Autodesk Inventor part; units mm, degrees
ref_plane "YZ Plane" through (0, 0, 0) normal (1, 0, 0) x (0, 1, 0)
ref_plane "XZ Plane" through (0, 0, 0) normal (0, 1, 0) x (-1, 0, 0)
ref_plane "XY Plane" through (0, 0, 0) normal (0, 0, 1) x (1, 0, 0)
sketch "Sketch1" plane through (0, 0, 0) normal (0, 0, 1) x (1, 0, 0)
  line L0 (-70, -100) -> (70, -100)
  line L1 (70, -100) -> (70, 100)
  line L2 (70, 100) -> (-70, 100)
  line L3 (-70, 100) -> (-70, -100)
  line L4 (-70, -100) -> (70, 100) construction
  line L5 (70, -100) -> (-70, 100) construction
  point P0 (0, 0)
  dimension "d154" = 140
  dimension "d155" = 200
extrude "Plate5" add sketch "Sketch1" along normal blind 2
sketch "Sketch7" plane through (68, -100, 2) normal (1, 0, 0) x (0, 1, 0)
  line L0 (200, 0) -> (0, 0)
  line L1 (0, 0) -> (0, -30)
  line L2 (0, -30) -> (200, -30)
  line L3 (200, -30) -> (200, 0)
edge flange "Flange3" height 30 angle 90 thickness 2 bend radius 2.75 thickness toward (1, 0, 0) relief round relief width 2 relief depth 1 corner gap 2.75 corner form 0 edges at (70, 0, 0) (-70, 0, 0) wall of the first edge with corners at (68, 100, 2) (68, -100, 2) (68, -100, -28) (68, 100, -28)
bend "Bend3"
corner "Corner3"
sketch "Sketch8" plane through (-68, -100, -26) normal (0, 0, -1) x (-1, 0, 0)
  line L0 (0, 200) -> (0, 0)
  line L1 (0, 0) -> (35, 0)
  line L2 (35, 0) -> (35, 200)
  line L3 (35, 200) -> (0, 200)
edge flange "Flange4" height 35 angle 90 thickness 2 bend radius 2.75 thickness toward (0, 0, -1) relief round relief width 2 relief depth 1 corner gap 2.75 corner form 0 edges at (-70, 0, -28) (70, 0, -28) wall of the first edge with corners at (-68, 100, -26) (-68, -100, -26) (-103, -100, -26) (-103, 100, -26)
bend "Bend4"
corner "Corner4"
sketch "Sketch9" plane through (-103, -100, -26) normal (0, 0, 1) x (1, 0, 0)
  line L0 (30.25, 0) -> (30.25, 200)
  line L1 (30.25, 200) -> (0, 200)
  line L2 (0, 200) -> (0, 0)
  line L3 (30.25, 0) -> (0, 0)
  circle A0 centre (10, 190) radius 5.5
  circle A1 centre (10, 10) radius 5.5
  point P0 (103, 100)
  dimension "d177" = 11
  dimension "d178" = 10
  dimension "d179" = 10
  dimension "d180" = 10
extrude "Cut1" cut sketch "Sketch9" against normal blind 2 contours A0 | A1
mirror "Mirror1" about plane through (0, 0, 0) normal (1, 0, 0) of "Cut1"
fillet "Corner Round2" radius 6 4 edges at (-103, 100, -27) (-103, -100, -27) (103, 100, -27) (103, -100, -27)
sketch "Sketch10" plane through (0, 0, 2) normal (0, 0, 1) x (1, 0, 0)
  circle A0 centre (-45, 56) radius 4
  line L0 (-45, 56) -> (45, 56) construction
  line L1 (45, 56) -> (45, -56) construction
  line L2 (45, -56) -> (-45, -56) construction
  line L3 (-45, -56) -> (-45, 56) construction
  circle A1 centre (45, 56) radius 4
  circle A2 centre (45, -56) radius 4
  circle A3 centre (-45, -56) radius 4
  point P0 (0, 0)
  point P1 (0, 56)
  point P2 (45, 0)
  dimension "d185" = 8
  dimension "d186" = 90
  dimension "d187" = 112
extrude "Cut2" cut sketch "Sketch10" against normal blind 2
properties part number "TKS mixer support" material "Stainless Steel"
Model file for the job. Use its own axes, mm. A direction names the side the tool comes from. Coordinates: 2 decimals unless noted, no trailing zeros. Write each loop counter-clockwise with the first axis right and the second up, starting at its lowest first coordinate (ties: lowest second). Pieces come first, ordered by that corner, then holes. Notation, with made-up numbers: (15.5, 59.5) - (51.5, 59.5) arc R24 ccw to (51.5, 73.5) - close; hole circle Ø1 at (21.5, 32). An arc over 180 degrees is marked (long way). One line per item, written item: value. Start each with the question number.
1. Slice it at A-A (z = -5.25). Write the cut outline in (x, y).
2. Probe line 1 (Y direction, x = -45, z = 0.55); line 2 (Y direction, x = 93, z = -26.7); line 3 (X direction, y = -57, z = -12). List the from-to ranges inside material, lowest first. Write a range as from..to.
3. Mould opens along X. For faces 3 (the cylindrical face through (68.645, -1.4, 0.572)), 4 (the cylindrical face through (-45.867, -59.905, 1.014)), 5 (the flat face through (-70, 1, -13)) say: released by +X, released by -X, zero draft, split by the parting line, or undercut.
4. Slice it at D-D (y = 56). Write the cut outline in (x, z), plus the area to 3 significant figures.
5. Slice it at C-C (y = -17.5). Write the cut outline in (x, z), plus the area to 3 significant figures.
6. Slice it at B-B (x = 45). Write the cut outline in (y, z).
7. Tool access for faces 1 (the flat face through (68, -1, -13)), 2 (the cylindrical face through (101.196, 98.289, -27.014)): list every direction of +Z, -Z, +X, -X, +Y, -Y with a clear straight run to the whole face (end or side of a thin tool).
8. Flat gauge pins, fed straight in: pin 1 (10 mm diameter, centred on x = 93, y = -90, fed in from -Z); pin 2 (16.5 mm diameter, centred on y = 32.5, z = -17.5, fed in from +X); pin 3 (6 mm diameter, centred on y = 39.5, z = -16.5, fed in from -X); pin 4 (24 mm diameter, centred on x = -83.5, y = 25, fed in from +Z). Where does each tip first touch, or does it go through?
Answers below:
1. outline: (-70, -100) - (-68, -100) - (-68, 100) - (-70, 100) - close; (68, -100) - (70, -100) - (70, 100) - (68, 100) - close
2. line 1: y = -100..-60, -52..52, 60..100
2. line 2: y = -100..-95.5, -84.5..84.5, 95.5..100
2. line 3: x = -70..-68, 68..70
3. face 3: released by +X
3. face 4: undercut
3. face 5: released by -X
4. outline: (-103, -28) - (-72.75, -28) arc R4.75 ccw to (-68, -23.25) - (-68, -2.75) arc R2.75 cw to (-65.25, 0) - (-49, 0) - (-49, 2) - (-65.25, 2) arc R4.75 ccw to (-70, -2.75) - (-70, -23.25) arc R2.75 cw to (-72.75, -26) - (-103, -26) - close; (-41, 0) - (41, 0) - (41, 2) - (-41, 2) - close; (49, 0) - (65.25, 0) arc R2.75 cw to (68, -2.75) - (68, -23.25) arc R4.75 ccw to (72.75, -28) - (103, -28) - (103, -26) - (72.75, -26) arc R2.75 cw to (70, -23.25) - (70, -2.75) arc R4.75 ccw to (65.25, 2) - (49, 2) - close
4. area: 479 mm^2
5. outline: (-103, -28) - (-72.75, -28) arc R4.75 ccw to (-68, -23.25) - (-68, -2.75) arc R2.75 cw to (-65.25, 0) - (65.25, 0) arc R2.75 cw to (68, -2.75) - (68, -23.25) arc R4.75 ccw to (72.75, -28) - (103, -28) - (103, -26) - (72.75, -26) arc R2.75 cw to (70, -23.25) - (70, -2.75) arc R4.75 ccw to (65.25, 2) - (-65.25, 2) arc R4.75 ccw to (-70, -2.75) - (-70, -23.25) arc R2.75 cw to (-72.75, -26) - (-103, -26) - close
5. area: 511 mm^2
6. outline: (-100, 0) - (-60, 0) - (-60, 2) - (-100, 2) - close; (-52, 0) - (52, 0) - (52, 2) - (-52, 2) - close; (60, 0) - (100, 0) - (100, 2) - (60, 2) - close
7. face 1: -Z, +Y, -Y
7. face 2: +Z, -Z, +X, +Y
8. pin 1: passes through
8. pin 2: stops at x = 71.6
8. pin 3: stops at x = -70
8. pin 4: stops at z = -25.7
